```python
from build123d import *

# Parameters (mm, degrees)
ESBO_O1_W                = 143.01
ESBO_O1_H                = 54
RESSALTO_EXTRUS_O1_DEPTH = 10
ESBO_O14_W               = 2.7
ESBO_O14_H               = 57.87
RESSALTO_EXTRUS_O3_DEPTH = 143.01
ESBO_O2_R                = 16
CIRCULO_ROLAMENTO_DEPTH  = 19
ESBO_O7_R                = 10
CORTE_EXTRUS_O3_DEPTH    = 19
ESBO_O8_W                = 143.01
ESBO_O8_H                = 3.87
RESSALTO_EXTRUS_O2_DEPTH = 10
ESBO_O22_W               = 143.01
ESBO_O22_H               = 3
RESSALTO_EXTRUS_O4_DEPTH = 12.7
ESBO_O12_R               = 2.5
CORTE_EXTRUS_O6_DEPTH    = 17
CORTE_EXTRUS_O15_REACH   = 80.913
ESBO_O9_R                = 2.568489929
ESBO_O9_R_2              = 2.65
CORTE_EXTRUS_O16_REACH   = 96.436
ESBO_O23_R               = 2.5


with BuildPart() as part:
    # Esboço1 → Ressalto-extrusão1 (new body)
    with BuildSketch(Plane.XY):
        Rectangle(ESBO_O1_W, ESBO_O1_H)
    extrude(amount=RESSALTO_EXTRUS_O1_DEPTH)

    # Esboço14 → Ressalto-extrusão3 (add)
    with BuildSketch(Plane.ZY.offset(71.505)):
        with Locations((-1.35, -1.935)):
            Rectangle(ESBO_O14_W, ESBO_O14_H)
    extrude(amount=-RESSALTO_EXTRUS_O3_DEPTH)

    # Esboço2 → Circulo rolamento (cut)
    with BuildSketch(Plane.XY.offset(10)):
        Circle(ESBO_O2_R)
    extrude(amount=-CIRCULO_ROLAMENTO_DEPTH, mode=Mode.SUBTRACT)

    # Esboço7 → Corte-extrusão3 (cut)
    with BuildSketch(Plane.XY.offset(10)):
        with Locations(Location((-44.465, 0, 0), (0, 0, 90))):
            Circle(ESBO_O7_R)
        with Locations((44.465, 0)):
            Circle(ESBO_O7_R)
    extrude(amount=-CORTE_EXTRUS_O3_DEPTH, mode=Mode.SUBTRACT)

    # Esboço8 → Ressalto-extrusão2 (add)
    with BuildSketch(Plane.XY.offset(10)):
        with Locations((0, -28.935)):
            Rectangle(ESBO_O8_W, ESBO_O8_H)
    extrude(amount=-RESSALTO_EXTRUS_O2_DEPTH)

    # Esboço22 → Ressalto-extrusão4 (add)
    with BuildSketch(Plane.XY.offset(10)):
        with Locations((0, 28.5)):
            Rectangle(ESBO_O22_W, ESBO_O22_H)
    extrude(amount=-RESSALTO_EXTRUS_O4_DEPTH)

    # Esboço12 → Corte-extrusão6 (cut)
    with BuildSketch(Plane.XZ.offset(30.87)):
        with Locations(Location((-61.505, 3.65, 0), (0, 0, 270))):
            Circle(ESBO_O12_R)
        with Locations(Location((33.505, 3.65, 0), (0, 0, 90))):
            Circle(ESBO_O12_R)
        with Locations(Location((0, 3.65, 0), (0, 0, 270))):
            Circle(ESBO_O12_R)
        with Locations(Location((-33.505, 3.65, 0), (0, 0, 270))):
            Circle(ESBO_O12_R)
        with Locations(Location((61.505, 3.65, 0), (0, 0, 90))):
            Circle(ESBO_O12_R)
    extrude(amount=-CORTE_EXTRUS_O6_DEPTH, mode=Mode.SUBTRACT)

    # Esboço9 → Corte-extrusão15 (cut, up to next)
    with BuildSketch(Plane.XY.offset(10), mode=Mode.PRIVATE) as corte_extrus_o15_sk1:
        with Locations((23.3, -23.3)):
            Circle(ESBO_O9_R)
    corte_extrus_o15_tool1 = extrude(corte_extrus_o15_sk1.sketch, amount=-CORTE_EXTRUS_O15_REACH, mode=Mode.PRIVATE) & part.part
    # Esboço9 → Corte-extrusão15 (cut, up to next)
    with BuildSketch(Plane.XY.offset(10), mode=Mode.PRIVATE) as corte_extrus_o15_sk2:
        with Locations((23.3, 23.3)):
            Circle(ESBO_O9_R_2)
    corte_extrus_o15_tool2 = extrude(corte_extrus_o15_sk2.sketch, amount=-CORTE_EXTRUS_O15_REACH, mode=Mode.PRIVATE) & part.part
    # Esboço9 → Corte-extrusão15 (cut, up to next)
    with BuildSketch(Plane.XY.offset(10), mode=Mode.PRIVATE) as corte_extrus_o15_sk3:
        with Locations((-23.3, -23.3)):
            Circle(ESBO_O9_R_2)
    corte_extrus_o15_tool3 = extrude(corte_extrus_o15_sk3.sketch, amount=-CORTE_EXTRUS_O15_REACH, mode=Mode.PRIVATE) & part.part
    # Esboço9 → Corte-extrusão15 (cut, up to next)
    with BuildSketch(Plane.XY.offset(10), mode=Mode.PRIVATE) as corte_extrus_o15_sk4:
        with Locations((-23.3, 23.3)):
            Circle(ESBO_O9_R_2)
    corte_extrus_o15_tool4 = extrude(corte_extrus_o15_sk4.sketch, amount=-CORTE_EXTRUS_O15_REACH, mode=Mode.PRIVATE) & part.part
    add(corte_extrus_o15_tool1.solids().sort_by_distance((23.3, -23.3, 10))[0], mode=Mode.SUBTRACT)
    add(corte_extrus_o15_tool2.solids().sort_by_distance((23.3, 23.3, 10))[0], mode=Mode.SUBTRACT)
    add(corte_extrus_o15_tool3.solids().sort_by_distance((-23.3, -23.3, 10))[0], mode=Mode.SUBTRACT)
    add(corte_extrus_o15_tool4.solids().sort_by_distance((-23.3, 23.3, 10))[0], mode=Mode.SUBTRACT)

    # Esboço23 → Corte-extrusão16 (cut, up to next)
    with BuildSketch(Plane(origin=(0, 30, 0), x_dir=(1, 0, 0), z_dir=(0, 1, 0)), mode=Mode.PRIVATE) as corte_extrus_o16_sk1:
        with Locations(Location((-44.505, -3.65, 0), (0, 0, 270))):
            Circle(ESBO_O23_R)
    corte_extrus_o16_tool1 = extrude(corte_extrus_o16_sk1.sketch, amount=-CORTE_EXTRUS_O16_REACH, mode=Mode.PRIVATE) & part.part
    # Esboço23 → Corte-extrusão16 (cut, up to next)
    with BuildSketch(Plane(origin=(0, 30, 0), x_dir=(1, 0, 0), z_dir=(0, 1, 0)), mode=Mode.PRIVATE) as corte_extrus_o16_sk2:
        with Locations(Location((44.505, -3.65, 0), (0, 0, 270))):
            Circle(ESBO_O23_R)
    corte_extrus_o16_tool2 = extrude(corte_extrus_o16_sk2.sketch, amount=-CORTE_EXTRUS_O16_REACH, mode=Mode.PRIVATE) & part.part
    add(corte_extrus_o16_tool1.solids().sort_by_distance((-44.505, 30, 3.65))[0], mode=Mode.SUBTRACT)
    add(corte_extrus_o16_tool2.solids().sort_by_distance((44.505, 30, 3.65))[0], mode=Mode.SUBTRACT)


solid = part.part
```
For this review, take the finished solid that the model builds, in its own axes (mm). A direction names the side the tool comes from. Round coordinates to 2 decimals unless told otherwise and drop trailing zeros. Write each loop counter-clockwise with the first axis right and the second up, starting at its lowest first coordinate (ties: lowest second). Pieces come first, ordered by that corner, then holes. Notation, with made-up numbers: (78.25, -18.75) -> (121.25, -18.75) arc R28 ccw to (121.25, 9.25) -> close; hole circle Ø4 at (-32, -36). An arc over 180 degrees is marked (long way). Use one line per item in the form item = value.
Q1. Consider section A-A (x = -23.3). State the section outline as (y, z) points.
Resolved:
outline = (-30.87, -2.7) -> (-25.95, -2.7) -> (-25.95, 10) -> (-30.87, 10) -> close; (-20.65, -2.7) -> (20.65, -2.7) -> (20.65, 10) -> (-20.65, 10) -> close; (25.95, -2.7) -> (30, -2.7) -> (30, 10) -> (25.95, 10) -> close
Q2. To check wall thickness, follow probe 1 along X at (y, z) = (-27, 3.65) (3 decimals); probe 2 along X at (y, z) = (-25, 8.75) (3 decimals); probe 3 along X at (y, z) = (-5, 6) (3 decimals). State the ranges of each line that lie inside material, in increasing order. Write a range as from..to.
Resolved:
probe_1 = -71.505..-64.005, -59.005..-36.005, -31.005..-2.5, 2.5..31.005, 36.005..59.005, 64.005..71.505
probe_2 = -71.505..-25.333, -21.267..21.375, 25.225..71.505
probe_3 = -71.505..-53.125, -35.805..-15.199, 15.199..35.805, 53.125..71.505
Q3. Machinability: for faces 5 (the cylindrical face through (46.984, 19.978, 3.325)), 6 (the cylindrical face through (-54.38, -1.3, 3.74)), 7 (the cylindrical face through (-35.946, -22.489, 4.192)), which of the approach directions +Z, -Z, +X, -X, +Y, -Y give a long, thin tool a straight path to every point of the face, cutting with its end or side? Answer none if there is none.
Resolved:
face_5 = +Y
face_6 = +Z, -Z
face_7 = -Y
Q4. Consider section C-C (y = 23.3). State the section outline as (x, z) points (3 decimals), then the cut area to 3 significant figures.
Resolved:
outline = (-71.505, -2.7) -> (-25.95, -2.7) -> (-25.95, 10) -> (-71.505, 10) -> close; (-20.65, -2.7) -> (20.65, -2.7) -> (20.65, 10) -> (-20.65, 10) -> close; (25.95, -2.7) -> (71.505, -2.7) -> (71.505, 10) -> (25.95, 10) -> close; hole circle Ø5 at (-44.505, 3.65); hole circle Ø5 at (44.505, 3.65)
area = 1,640 mm²
Q5. Consider section D-D (x = 52.5). State the section outline as (y, z) points.
Resolved:
outline = (-30.87, -2.7) -> (-5.95, -2.7) -> (-5.95, 10) -> (-30.87, 10) -> close; (5.95, -2.7) -> (30, -2.7) -> (30, 10) -> (5.95, 10) -> close
Q6. Consider section B-B (y = 0). State the section outline as (x, z) points (3 decimals), then the cut area to 3 significant figures.
Resolved:
outline = (-71.505, -2.7) -> (-54.465, -2.7) -> (-54.465, 10) -> (-71.505, 10) -> close; (-34.465, -2.7) -> (-16, -2.7) -> (-16, 10) -> (-34.465, 10) -> close; (16, -2.7) -> (34.465, -2.7) -> (34.465, 10) -> (16, 10) -> close; (54.465, -2.7) -> (71.505, -2.7) -> (71.505, 10) -> (54.465, 10) -> close
area = 902 mm²
Q7. The part is to be moulded in two halves that separate along Y. For faces 1 (the flat face through (-61, -13.87, 4)), 2 (the flat face through (-71.505, -1, 4)), 3 (the cylindrical face through (-23.87, 20.71, 3.74)), 4 (the cylindrical face through (21.26, -24.86, 3.74)), say which applies: released by +Y, released by -Y, zero draft, split by the parting line, or undercut.
Resolved:
face_1 = released by -Y
face_2 = zero draft
face_3 = undercut
face_4 = undercut
Q8. Clearance check with flat-ended pins moving along their axes: pin 1 Ø4 at (x, z) = (61.505, 3.65) entering from -Y; pin 2 Ø2.5 at (x, z) = (33, 5) entering from -Y; pin 3 Ø1.5 at (x, z) = (44.5, 2) entering from +Y. State where each tip first meets the part, or that it passes through.
Resolved:
pin_1 = -13.87
pin_2 = -30.87
pin_3 = -9.97
